from build123d import *

# Parameters (mm, degrees)
SKETCH_1_R      = 0.5
EXTRUDE_2_DEPTH = 1


with BuildPart() as part:
    # Эскиз1 → Бобышка-Вытянуть2 (new body)
    with BuildSketch(Plane(origin=(0, 0, 0), x_dir=(1, 0, 0), z_dir=(0, 1, 0))):
        Polygon((25, -23.1), (25, -19), (23.1, -19), (23.1, -17), (25, -17), (25, -13), (23.1, -13), (23.1, -11), (25, -11), (25, -7), (23.1, -7), (23.1, -5), (25, -5), (25, -1), (23.1, -1), (23.1, 1), (25, 1), (25, 5), (23.1, 5), (23.1, 7), (25, 7), (25, 11), (23.1, 11), (23.1, 13), (25, 13), (25, 17), (23.1, 17), (23.1, 19), (25, 19), (25, 25), (19, 25), (19, 23.1), (17, 23.1), (17, 25), (13, 25), (13, 23.1), (11, 23.1), (11, 25), (7, 25), (7, 23.1), (5, 23.1), (5, 25), (1, 25), (1, 23.1), (-1, 23.1), (-1, 25), (-5, 25), (-5, 23.1), (-7, 23.1), (-7, 25), (-11, 25), (-11, 23.1), (-13, 23.1), (-13, 25), (-17, 25), (-17, 23.1), (-19, 23.1), (-19, 25), (-23.1, 25), (-23.1, 19), (-25, 19), (-25, 17), (-23.1, 17), (-23.1, 13), (-25, 13), (-25, 11), (-23.1, 11), (-23.1, 7), (-25, 7), (-25, 5), (-23.1, 5), (-23.1, 1), (-25, 1), (-25, -1), (-23.1, -1), (-23.1, -5), (-25, -5), (-25, -7), (-23.1, -7), (-23.1, -11), (-25, -11), (-25, -13), (-23.1, -13), (-23.1, -17), (-25, -17), (-25, -19), (-23.1, -19), (-23.1, -23.1), (-19, -23.1), (-19, -25), (-17, -25), (-17, -23.1), (-13, -23.1), (-13, -25), (-11, -25), (-11, -23.1), (-7, -23.1), (-7, -25), (-5, -25), (-5, -23.1), (-1, -23.1), (-1, -25), (1, -25), (1, -23.1), (5, -23.1), (5, -25), (7, -25), (7, -23.1), (11, -23.1), (11, -25), (13, -25), (13, -23.1), (17, -23.1), (17, -25), (19, -25), (19, -23.1), align=None)
        with Locations(Location((18, -24.05, 0), (0, 0, 270))):
            Circle(SKETCH_1_R, mode=Mode.SUBTRACT)
        with Locations(Location((12, -24.05, 0), (0, 0, 270))):
            Circle(SKETCH_1_R, mode=Mode.SUBTRACT)
        with Locations(Location((6, -24.05, 0), (0, 0, 270))):
            Circle(SKETCH_1_R, mode=Mode.SUBTRACT)
        with Locations(Location((0, -24.05, 0), (0, 0, 270))):
            Circle(SKETCH_1_R, mode=Mode.SUBTRACT)
        with Locations(Location((-6, -24.05, 0), (0, 0, 270))):
            Circle(SKETCH_1_R, mode=Mode.SUBTRACT)
        with Locations(Location((-12, -24.05, 0), (0, 0, 270))):
            Circle(SKETCH_1_R, mode=Mode.SUBTRACT)
        with Locations(Location((-18, -24.05, 0), (0, 0, 270))):
            Circle(SKETCH_1_R, mode=Mode.SUBTRACT)
        with Locations(Location((-24.05, -18, 0), (0, 0, 270))):
            Circle(SKETCH_1_R, mode=Mode.SUBTRACT)
        with Locations(Location((-24.05, -12, 0), (0, 0, 270))):
            Circle(SKETCH_1_R, mode=Mode.SUBTRACT)
        with Locations(Location((-24.05, -6, 0), (0, 0, 270))):
            Circle(SKETCH_1_R, mode=Mode.SUBTRACT)
        with Locations(Location((-24.05, 0, 0), (0, 0, 270))):
            Circle(SKETCH_1_R, mode=Mode.SUBTRACT)
        with Locations(Location((-24.05, 6, 0), (0, 0, 270))):
            Circle(SKETCH_1_R, mode=Mode.SUBTRACT)
        with Locations(Location((-24.05, 12, 0), (0, 0, 270))):
            Circle(SKETCH_1_R, mode=Mode.SUBTRACT)
        with Locations(Location((-24.05, 18, 0), (0, 0, 270))):
            Circle(SKETCH_1_R, mode=Mode.SUBTRACT)
    extrude(amount=EXTRUDE_2_DEPTH)


solid = part.part
The listing builds one solid part. Answer for the finished solid, in the listing's coordinates (mm). Give positions to 0.01 mm unless a question says otherwise; leave off trailing zeros. Write each loop counter-clockwise with the first axis right and the second up, starting at its lowest first coordinate (ties: lowest second). Pieces come first, ordered by that corner, then holes. Notation, with made-up numbers: (73, -36.5) - (86, -36.5) arc R13 cw to (86, -25.5) - close; hole circle Ø10 at (43.25, -29). An arc over 180 degrees is marked (long way). One line per question, with ' | ' between items. Start each with the question number.
1. Section C-C, the plane z = 14 is taken. Determine the outline of the cut face in (x, y).
2. Given P1, Ø0.5, axis at y = 0.5, z = -24, coming from the -X side; P2, Ø0.5, axis at x = 6.5, y = 0.5, coming from the -Z side; P3, Ø0.5, axis at x = -24.5, y = 0.5, coming from the +Z side, each flat-ended and moving along its own axis, determine where each tip first touches the part or whether it passes through.
3. Straight lines are drawn through the part: line 1 (X direction, y = 0.65, z = -12); line 2 (X direction, y = 0.25, z = -4.5); line 3 (Z direction, x = -16.5, y = 0.4). For each, find the intervals that lie inside material, in ascending order.
4. Section A-A, the plane y = 0.15 is taken. Count the separate pieces of the cut face and the enclosed holes in it, then the cut area to 3 significant figures.
5. Section B-B, the plane x = -2 is taken. Determine the outline of the cut face in (y, z).
Result:
1) outline: (-23.1, 0) - (25, 0) - (25, 1) - (-23.1, 1) - close
2) P1: stops at x = -23.1 | P2: stops at z = -23.1 | P3: stops at z = 19
3) line 1: x = -25 to -24.55, -23.55 to 23.1 | line 2: x = -23.1 to 25 | line 3: z = -25 to 23.1
4) separate pieces: 1 | enclosed holes: 14 | area: 2,300 mm2
5) outline: (0, -25) - (1, -25) - (1, 23.1) - (0, 23.1) - close
